For this review, take the finished solid that the model builds, in its own axes (mm). Face numbers are marked on the shaded views. A direction names the side the tool comes from. Coordinates: 2 decimals unless noted, no trailing zeros. Order: outer loops, then holes, each group sorted by start corner. A loop starts at its lowest first (then second) coordinate and runs counter-clockwise, first axis right, second up.
from build123d import *

# Parameters (mm, degrees)
BOSS_EXTRUDE1_DEPTH = 2.5
SKETCH2_W           = 0.55
SKETCH2_H           = 0.55
BOSS_EXTRUDE2_DEPTH = 6


with BuildPart() as part:
    # Sketch1 → Boss-Extrude1 (new body)
    with BuildSketch(Plane.XY):
        Polygon((0, 0), (0, 4), (0.5, 4.504083326), (2.04, 4.504083326), (2.544083326, 4.004083326), (3.044083326, 4.508166653), (4.584083326, 4.508166653), (5.088166653, 4.008166653), (5.590208299, 4.510216636), (7.130195513, 4.51649212), (7.632245496, 4.014450474), (8.134287142, 4.516500457), (9.674274356, 4.522775941), (10.176324339, 4.020734295), (10.674266053, 4.526850931), (12.214253267, 4.533126415), (12.720369903, 4.035184701), (13.218311617, 4.541301337), (14.758298831, 4.547576821), (15.264415467, 4.049635107), (15.28891529, 0.041535012), (14.786873643, -0.460514971), (13.24688643, -0.466790455), (12.740769794, 0.031151259), (12.238728147, -0.470898724), (10.698740934, -0.477174208), (10.192624298, 0.020767506), (9.690582651, -0.481282477), (8.150595438, -0.487557961), (7.644478802, 0.010383753), (7.142437155, -0.49166623), (5.602449942, -0.497941714), (5.096333306, 0), (4.592249979, -0.5), (3.052249979, -0.5), (2.548166653, 0), (2.044083326, -0.5), (0.504083326, -0.5), align=None)
    extrude(amount=BOSS_EXTRUDE1_DEPTH)

    # Sketch2 → Boss-Extrude2 (add)
    with BuildSketch(Plane.XY):
        with Locations((6.375, 0.705)):
            Rectangle(SKETCH2_W, SKETCH2_H)
        with Locations((3.825, 0.705)):
            Rectangle(SKETCH2_W, SKETCH2_H)
        with Locations((14.025, 0.705)):
            Rectangle(SKETCH2_W, SKETCH2_H)
        with Locations((14.025, 3.305)):
            Rectangle(SKETCH2_W, SKETCH2_H)
        with Locations((8.925, 0.705)):
            Rectangle(SKETCH2_W, SKETCH2_H)
        with Locations((1.275, 0.705)):
            Rectangle(SKETCH2_W, SKETCH2_H)
        with Locations((11.475, 0.705)):
            Rectangle(SKETCH2_W, SKETCH2_H)
        with Locations((1.275, 3.305)):
            Rectangle(SKETCH2_W, SKETCH2_H)
    extrude(amount=-BOSS_EXTRUDE2_DEPTH)


solid = part.part
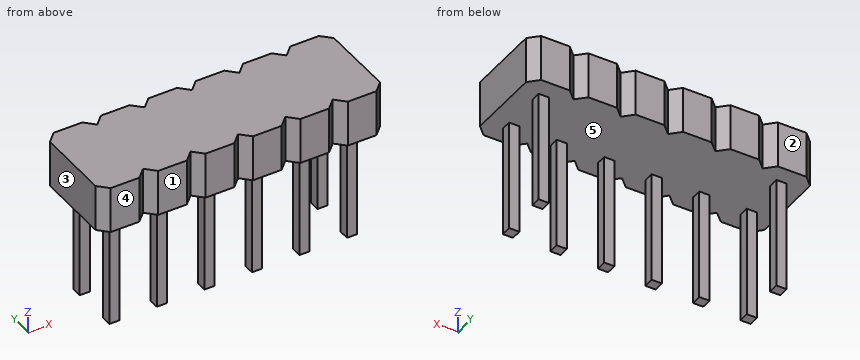
1. Take a section at D-D, the plane y = 0.2. Give the boundary of the cut face in (x, z).
Answer below:
outline: (0, 0) - (15.29, 0) - (15.29, 2.5) - (0, 2.5) - close
2. Clearance check with flat-ended pins moving along their axes: pin 1 Ø4 at (x, z) = (12, -0.5) entering from +Y; pin 2 Ø0.6 at (x, z) = (11.5, -2) entering from +Y; pin 3 Ø0.6 at (x, z) = (1.5, -2.5) entering from -Y. State where each tip first meets the part, or that it passes through.
Answer below:
pin 1: stops at y = 4.54
pin 2: stops at y = 0.98
pin 3: stops at y = 0.43
3. Take a section at C-C, the plane y = 2.6. Give the boundary of the cut face in (x, z), plus the area to 3 significant figures.
Answer below:
outline: (0, 0) - (15.27, 0) - (15.27, 2.5) - (0, 2.5) - close
area: 38.2 mm2
4. The part is to be moulded in two halves that separate along X. For the marked faces 3, 4 and 5, say which applies: +X half, -X half, draft (parallel to the pull), parting line (faces both ways), or undercut.
Answer below:
face 3: -X half
face 4: draft
face 5: undercut
5. Machinability: for the marked faces 1 and 2, which of the approach directions +Z, -Z, +X, -X, +Y, -Y give a long, thin tool a straight path to every point of the face, cutting with its end or side? Answer none if there is none.
Answer below:
face 1: +Z, -Z, +X, -X, -Y
face 2: +Z, -Z, -X, +Y
6. Take a section at B-B, the plane x = 3.75. Give the boundary of the cut face in (y, z), plus the area to 3 significant figures.
Answer below:
outline: (-0.5, 0) - (0.43, 0) - (0.43, -6) - (0.98, -6) - (0.98, 0) - (4.51, 0) - (4.51, 2.5) - (-0.5, 2.5) - close
area: 15.8 mm2
7. To check wall thickness, follow L1, parallel to X at y = 0.7, z = -0.5; L2, parallel to X at y = 3.2, z = -4.75; L3, parallel to Z at x = 9.75, y = 3.15. State the ranges of each line that lie inside material, in increasing order.
Answer below:
L1: x = 1 to 1.55, 3.55 to 4.1, 6.1 to 6.65, 8.65 to 9.2, 11.2 to 11.75, 13.75 to 14.3
L2: x = 1 to 1.55, 13.75 to 14.3
L3: z = 0 to 2.5
8. Take a section at A-A, the plane z = -2.25. Give the number of separate pieces and of enclosed holes in the cut face, plus the area to 3 significant figures.
Answer below:
separate pieces: 8
enclosed holes: 0
area: 2.42 mm2
